```python
from build123d import *
from build123d.topology import SkipClean

# Parameters (mm, degrees)
IZIM2_R               = 3
KES_EKSTR_ZYON1_DEPTH = 20
PAH1_SIZE             = 1
PAH2_SIZE             = 1


with BuildPart() as part:
    # Çizim1 → Döndür2 (revolve)
    with SkipClean():  # the faces are left unmerged after this step: merging them gives an invalid solid
        with BuildSketch(Plane.XY):
            with BuildLine():
                ThreePointArc((14.75, 0), (10.429825023, 10.429825023), (0, 14.75))
                Line((0, 14.75), (0, -14.75))
                ThreePointArc((0, -14.75), (10.429825023, -10.429825023), (14.75, 0))
            make_face()
            with BuildLine():
                Line((0, -14.75), (0, 14.75))
                ThreePointArc((0, 14.75), (-14.75, 0), (0, -14.75))
            make_face()
        revolve(axis=Axis((0, 19.521191609, 0), (0, -1, 0)))

    # Çizim2 → Kes-Ekstrüzyon1 (cut)
    with BuildSketch(Plane(origin=(0, 14.75, 0), x_dir=(1, 0, 0), z_dir=(0, 1, 0))):
        with Locations(Location((0, 0, 0), (0, 0, 270))):
            Circle(IZIM2_R)
    extrude(amount=-KES_EKSTR_ZYON1_DEPTH, mode=Mode.SUBTRACT)

    # Pah1
    # the kernel refuses this chamfer: 1, 0.845674781 mm, written as the material it takes off along each edge
    with BuildSketch(Plane(origin=(0, 14.441693114, 0), x_dir=(0, 0, 1), z_dir=(1, 0, 0))) as pah1_piece_1:
        with BuildLine():
            Line((3.808218247, 0.191781753), (3, PAH1_SIZE))
            Line((3, PAH1_SIZE), (3, 0))
            ThreePointArc((3, 0), (3.415662232, 0.092625147), (3.808218247, 0.191781753))
        make_face()
    revolve(axis=Axis((0, 14.441693114, 0), (0, -1, 0)), revolution_arc=270, mode=Mode.SUBTRACT)
    with BuildSketch(Plane(origin=(0, 14.441693114, 0), x_dir=(0, 0, 1), z_dir=(-1, 0, 0))) as pah1_piece_2:
        with BuildLine():
            Line((3.808218247, -0.191781753), (3, -PAH1_SIZE))
            Line((3, -PAH1_SIZE), (3, 0))
            ThreePointArc((3, 0), (3.415662232, -0.092625147), (3.808218247, -0.191781753))
        make_face()
    revolve(axis=Axis((0, 14.441693114, 0), (0, 1, 0)), revolution_arc=90, mode=Mode.SUBTRACT)

    # Pah2
    pah2_edges = [part.edges().sort_by_distance(p)[0] for p in [
        (0, -5.25, -3),
    ]]
    chamfer(pah2_edges, length=PAH2_SIZE)


solid = part.part
```
Check sheet for the modelled part. Datum: model origin and axes. Units: mm. Give positions to 0.01 mm unless a question says otherwise; leave off trailing zeros. Write each loop counter-clockwise with the first axis right and the second up, starting at its lowest first coordinate (ties: lowest second). Pieces come first, ordered by that corner, then holes.
Item 1: Cross-section at C-C (y = 6). Enter the section's corners in (x, z).
Item 2: Cross-section at D-D (z = 9). Enter the section's corners in (x, y), and give its area (3 significant figures).
Item 3: Draft check along X on faces 1 (the face through (0.9, 4.72, 2.86)), 2 (the face through (0, -5.25, 0)). Enter one of: released by +X, released by -X, zero draft, split by the parting line, or undercut.
Item 4: Scan lines: L1, parallel to X at y = 0, z = 0; L2, parallel to Z at x = 0, y = 1.25; L3, parallel to Z at x = 0, y = 4.5. Record each from-to range of solid material in increasing order.
Item 5: Cross-section at A-A (x = 0). Enter the section's corners in (y, z).
Item 6: Cross-section at B-B (z = 0). Enter the section's corners in (x, y).
Item 7: Gauge pin test, flat ends, axial feed: pin 1 (4.5 mm diameter, centred on x = -0.5, z = 0, fed in from +Y); pin 2 (10 mm diameter, centred on y = 1, z = 7.5, fed in from -X) (3 decimals); pin 3 (1 mm diameter, centred on x = 1.5, y = -5.5, fed in from +Z). Record the tip position at first contact, or that the pin passes through.
Report:
1. outline: circle Ø26.95 at (0, 0); hole circle Ø6 at (0, 0)
2. outline: circle Ø23.37 at (0, 0)
2. area: 429 mm2
3. face 1: undercut
3. face 2: undercut
4. L1: x = -14.75 to -3, 3 to 14.75
4. L2: z = -14.7 to -3, 3 to 14.7
4. L3: z = -14.05 to -3, 3 to 14.05
5. outline: (-5.25, -2) - (-5.25, 2) - (-4.25, 3) - (13.44, 3) - (14.25, 3.81) arc R14.75 ccw (long way) to (14.25, -3.81) - (13.44, -3) - (-4.25, -3) - close
6. outline: (-3.81, 14.25) arc R14.75 ccw (long way) to (3.81, 14.25) - (3, 13.44) - (3, -4.25) - (2, -5.25) - (-2, -5.25) - (-3, -4.25) - (-3, 13.44) - close
7. pin 1: stops at y = -4.5
7. pin 2: stops at x = -14.525
7. pin 3: stops at z = 13.8
